Answer from the drawing. Dimensions are ordinates in mm from the lowest x, y and z of the part. A direction names the side the tool comes from. Give positions to 0.01 mm unless a question says otherwise; leave off trailing zeros. Order: outer loops, then holes, each group sorted by start corner. A loop starts at its lowest first (then second) coordinate and runs counter-clockwise, first axis right, second up. Notation, with made-up numbers: (59.5, 47) - (93.5, 47) arc R19 ccw to (93.5, 60) - close; hole circle Ø2 at (36.5, -33.75). An arc over 180 degrees is marked (long way). Use a Markdown table: item, result. Add a question column.
1) Find section B-B, the plane z = 1.05. Determine the outline of the cut face in (x, y), plus the area to 3 significant figures.
2) Flat-ended cylindrical pins translate along their axes: pin 1 (0.9 mm diameter, centred on x = 30.5, z = 2, fed in from -Y); pin 2 (1.5 mm diameter, centred on x = 28.5, z = 1, fed in from +Y); pin 3 (0.9 mm diameter, centred on x = 20.5, z = 2, fed in from +Y). Find the tip coordinate at first contact, or state that the pin passes through.
3) Find section A-A, the plane y = 16. Determine the outline of the cut face in (x, z), plus the area to 3 significant figures.
4) Find section C-C, the plane x = 16.5. Determine the outline of the cut face in (y, z).
5) Straight lines are drawn through the part: line 1 (X direction, y = 4, z = 2.35); line 2 (X direction, y = 1.5, z = 1.5); line 3 (Y direction, x = 10, z = 2.4). For each, find the intervals that lie inside material, in ascending order.
6) For the marked faces 1, 2, 3 and 4, determine the directions among +Z, -Z, +X, -X, +Y, -Y from which every point of the face is accessible in a straight line to the end or side of a thin tool.
7) The mould has two halves that part along X. Classify the marked faces 5, 6 and 7: released by +X, released by -X, zero draft, split by the parting line, or undercut.
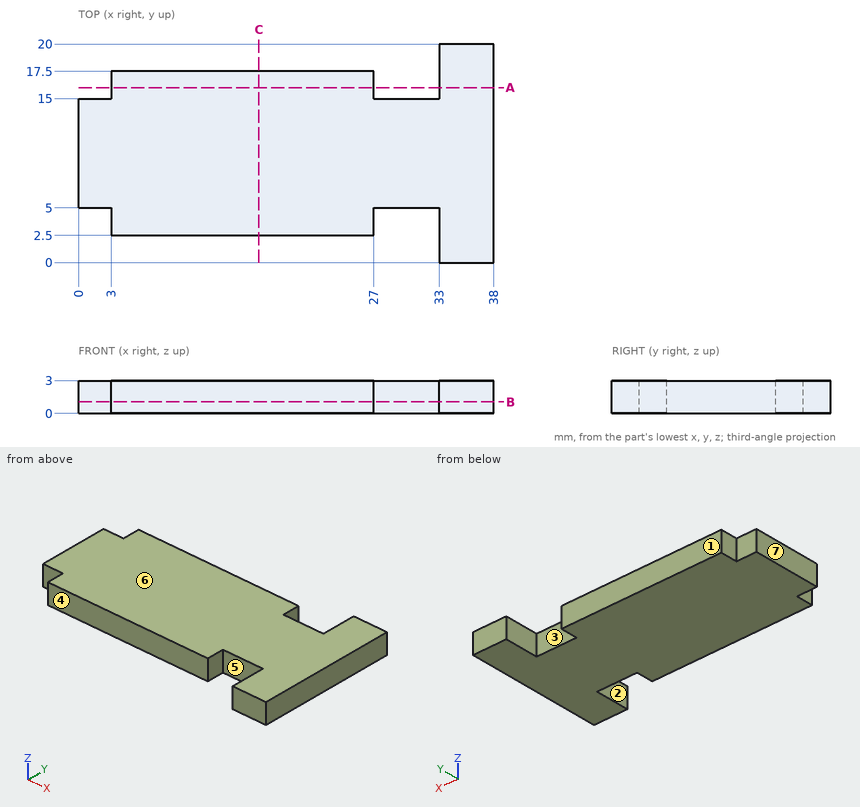
The answers:
| question | item | result |
|---|---|---|
| 1 | outline | (0, 5) - (3, 5) - (3, 2.5) - (27, 2.5) - (27, 5) - (33, 5) - (33, 0) - (38, 0) - (38, 20) - (33, 20) - (33, 15) - (27, 15) - (27, 17.5) - (3, 17.5) - (3, 15) - (0, 15) - close |
| 1 | area | 550 mm2 |
| 2 | pin 1 | y = 5 |
| 2 | pin 2 | y = 15 |
| 2 | pin 3 | y = 17.5 |
| 3 | outline | (3, 0) - (27, 0) - (27, 3) - (3, 3) - close; (33, 0) - (38, 0) - (38, 3) - (33, 3) - close |
| 3 | area | 87.0 mm2 |
| 4 | outline | (2.5, 0) - (17.5, 0) - (17.5, 3) - (2.5, 3) - close |
| 5 | line 1 | 3 to 27, 33 to 38 |
| 5 | line 2 | 33 to 38 |
| 5 | line 3 | 2.5 to 17.5 |
| 6 | face 1 | +Z, -Z, -X, +Y |
| 6 | face 2 | +Z, -Z, -Y |
| 6 | face 3 | +Z, -Z, +Y |
| 6 | face 4 | +Z, -Z, -X, -Y |
| 7 | face 5 | undercut |
| 7 | face 6 | zero draft |
| 7 | face 7 | released by -X |
